The figure shows three views and two pictorial views of one solid part (mm, origin at its lowest corner). Answer the questions. A direction names the side the tool comes from. Coordinates: 2 decimals unless noted, no trailing zeros. Loops run counter-clockwise (first coordinate to the right, second up) from the corner with the lowest first, then second, coordinate; pieces in that order, holes last. Notation, with made-up numbers: (-32.75, 35) -> (8.25, 35) arc R19 ccw to (8.25, 69) -> close; hole circle Ø6 at (16, 81). An arc over 180 degrees is marked (long way). Answer as a JSON object with one key per item and string values. Group by question number.
1) Section D-D, the plane y = 6.75 is taken. Give the vertices of the cut face in (x, z), plus the area to 3 significant figures.
2) Consider probe 1 along Z at (x, y) = (12, 1.95); probe 2 along Z at (x, y) = (3, 7); probe 3 along X at (y, z) = (4, 50). Determine where each line is inside the solid, lowest interval first. Write a range as [from, to].
3) Determine the mould class of the marked faces 1, 2 and 3 for opening direction X: released by +X, released by -X, zero draft, split by the parting line, or undercut.
4) Section C-C, the plane z = 55 is taken. Count the separate pieces of the cut face and the enclosed holes in it, plus the area to 3 significant figures.
5) Section A-A, the plane z = 62 is taken. Give the vertices of the cut face in (x, y), plus the area to 3 significant figures.
6) Section B-B, the plane x = 12 is taken. Give the vertices of the cut face in (y, z), plus the area to 3 significant figures.
7) A flat-ended cylindrical pin translates along its axis: P1, Ø1.5, axis at x = 40, y = 4, coming from the +Z side. Find the tip coordinate at first contact, or state that the pin passes through.
8) Which of the six approach directions +Z, -Z, +X, -X, +Y, -Y give full straight-line access (tool end or side, diameter ignored) to the marked faces 4 and 5?
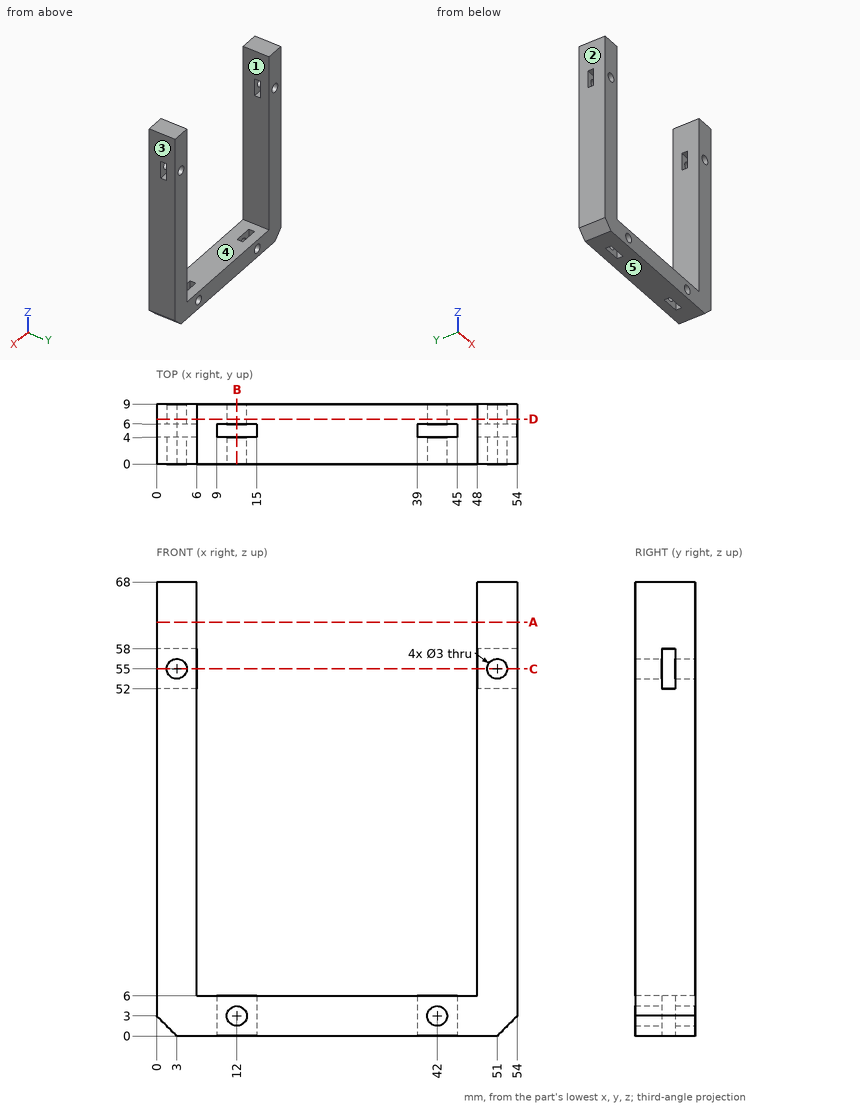
Determined:
{
 "1": {"outline": "(0, 3) -> (3, 0) -> (51, 0) -> (54, 3) -> (54, 68) -> (48, 68) -> (48, 6) -> (6, 6) -> (6, 68) -> (0, 68) -> close; hole circle Ø3 at (3, 55); hole circle Ø3 at (12, 3); hole circle Ø3 at (42, 3); hole circle Ø3 at (51, 55)", "area": "1,030 mm²"},
 "2": {"probe 1": "[0, 1.5], [4.5, 6]", "probe 2": "[0, 53.5], [56.5, 68]", "probe 3": "[0, 6], [48, 54]"},
 "3": {"face 1": "undercut", "face 2": "released by -X", "face 3": "released by +X"},
 "4": {"separate pieces": "8", "enclosed holes": "0", "area": "42.0 mm²"},
 "5": {"outline": "(0, 0) -> (6, 0) -> (6, 9) -> (0, 9) -> close; (48, 0) -> (54, 0) -> (54, 9) -> (48, 9) -> close", "area": "108 mm²"},
 "6": {"outline": "(0, 0) -> (4, 0) -> (4, 1.5) -> (0, 1.5) -> close; (0, 4.5) -> (4, 4.5) -> (4, 6) -> (0, 6) -> close; (6, 0) -> (9, 0) -> (9, 1.5) -> (6, 1.5) -> close; (6, 4.5) -> (9, 4.5) -> (9, 6) -> (6, 6) -> close", "area": "21.0 mm²"},
 "7": {"P1": "z = 6"},
 "8": {"face 4": "+Z, +Y, -Y", "face 5": "-Z, +X, -X, +Y, -Y"}
}
